Check sheet for the drawn part. Datum: minimum x, y, z corner. Units: mm. A direction names the side the tool comes from. Coordinates: 2 decimals unless noted, no trailing zeros. Loops run counter-clockwise (first coordinate to the right, second up) from the corner with the lowest first, then second, coordinate; pieces in that order, holes last. Notation, with made-up numbers: M 47.5,-17 L 83.5,-17 A26 cw 83.5,17 Z; hole C 68.5,19.5 d6. An arc over 180 degrees is marked long. Use CSV: the item, a comma, the result in double quotes. Start each with the question number.
(1) Section check B-B on y = 22. Record the cut outline in (x, z).
(2) Scan lines: line 1 (X direction, y = 53, z = 33); line 2 (X direction, y = 101.1, z = 25); line 3 (X direction, y = 100.55, z = 25). Record each from-to range of solid material in increasing order.
(3) Set-up check for the marked faces 4 and 5: record each of +Z, -Z, +X, -X, +Y, -Y from which the full face is reachable in a straight line by a thin tool's end or side.
(4) Section check A-A on x = 32. Record the cut outline in (y, z), and give its area (3 significant figures).
(5) Section check D-D on z = 5. Record the cut outline in (x, y).
(6) Section check C-C on x = 43. Record the cut outline in (y, z).
(7) Draft check along X on the marked faces 1, 2 and 3. Enter one of: pulls with the +X half, pulls with the -X half, needs draft (parallel to the pull), parting line crosses it, or undercut.
(8) Go/stop test with flat-tipped pins: pin 1 Ø2.5 at (x, z) = (21, 25) entering from -Y; pin 2 Ø1 at (x, z) = (10.5, 29) entering from -Y. Record where each tip stops, or that it passes through.
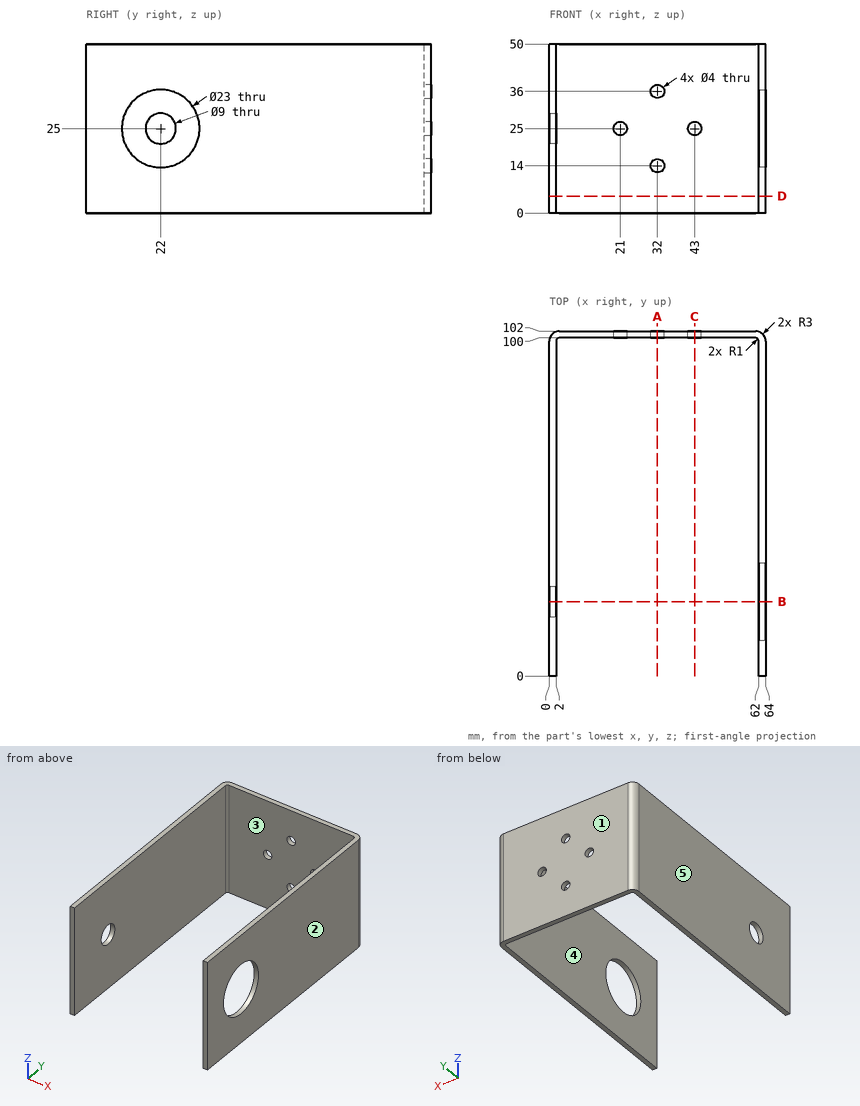
Outcome:
1,outline,"M 0,0 L 2,0 L 2,20.5 L 0,20.5 Z; M 0,29.5 L 2,29.5 L 2,50 L 0,50 Z; M 62,0 L 64,0 L 64,13.5 L 62,13.5 Z; M 62,36.5 L 64,36.5 L 64,50 L 62,50 Z"
2,line 1,"x = 0 to 2, 62 to 64"
2,line 2,"x = 0.86 to 19, 23 to 41, 45 to 63.14"
2,line 3,"x = 0.43 to 19, 23 to 41, 45 to 63.57"
3,face 4,"+Z, -Z, -Y"
3,face 5,"+Z, -Z, -X, +Y, -Y"
4,outline,"M 100,0 L 102,0 L 102,12 L 100,12 Z; M 100,16 L 102,16 L 102,34 L 100,34 Z; M 100,38 L 102,38 L 102,50 L 100,50 Z"
4,area,"84.0 mm²"
5,outline,"M 0,0 L 2,0 L 2,99 A1 cw 3,100 L 61,100 A1 cw 62,99 L 62,0 L 64,0 L 64,99 A3 ccw 61,102 L 3,102 A3 ccw 0,99 Z"
6,outline,"M 100,0 L 102,0 L 102,23 L 100,23 Z; M 100,27 L 102,27 L 102,50 L 100,50 Z"
7,face 1,"needs draft"
7,face 2,"pulls with the +X half"
7,face 3,"undercut"
8,pin 1,"passes through"
8,pin 2,"stops at y = 100"
